from build123d import *

# Parameters (mm, degrees)
F10_W     = 100
F10_H     = 100
F14_DEPTH = 35
F13_W     = 70
F13_H     = 70
F15_DEPTH = 65
F16_T     = -5
F21_D     = 25.4


# Not quite as in the source:
# - the program builds the solid bodies; features that only make, move or delete a surface that nothing else refers to are left out


with BuildPart() as f14:
    # F10 (on offset) → F14 (new body, through all)
    with BuildSketch(Plane.XZ.offset(-406.68448)):
        with Locations((37.5531539321, 417.7168309689)):
            Rectangle(F10_W, F10_H)
    extrude(amount=-F14_DEPTH)

    # F13 (on offset) → F15 (join, through all)
    with BuildSketch(Plane.XZ.offset(-506.68448)):
        with Locations((37.5531539321, 417.7168309689)):
            Rectangle(F13_W, F13_H)
    extrude(amount=F15_DEPTH)

    # F16
    f16_openings = [f14.faces().sort_by_distance(p)[0] for p in [
        (37.553154, 406.68448, 417.716831),
    ]]
    offset(amount=F16_T, openings=f16_openings, kind=Kind.INTERSECTION)

    # F21 (through all)
    with Locations(Plane.XZ.offset(-441.68448)):
        with Locations((37.5531539321, 417.7168309689)):
            Hole(F21_D / 2)


solid = f14.part
Work out the finished part from the listing and answer in its coordinate system (mm). A direction names the side the tool comes from. Give positions to 0.01 mm unless a question says otherwise; leave off trailing zeros. Write each loop counter-clockwise with the first axis right and the second up, starting at its lowest first coordinate (ties: lowest second). Pieces come first, ordered by that corner, then holes. Notation, with made-up numbers: (69.5, -37) - (89.5, -37) arc R36 cw to (89.5, 2) - close; hole circle Ø3 at (-31.75, 41.5). An arc over 180 degrees is marked (long way). One line per item, written item: value. Start each with the question number.
1. Given pin 1 (6 mm diameter, centred on x = 32, y = 493, fed in from -Z); pin 2 (12 mm diameter, centred on y = 469.5, z = 419.5, fed in from +X); pin 3 (1 mm diameter, centred on x = 1.5, z = 383.5, fed in from +Y), each flat-ended and moving along its own axis, determine where each tip first touches the part or whether it passes through.
2. Find section B-B (x = 38). Write down the section's boundary in (y, z).
3. Find section D-D (x = 71). Write down the section's boundary in (y, z), then the cut area to 3 significant figures.
4. Find section A-A (y = 484). Write down the section's boundary in (x, z), then the cut area to 3 significant figures.
5. Consider probe 1 along Z at (x, y) = (33, 460); probe 2 along X at (y, z) = (460, 437); probe 3 along Z at (x, y) = (22, 419.5). Determine where each line is inside the solid, lowest interval first.
6. Find section C-C (z = 385). Write down the section's boundary in (x, y).
7. For a pull along Z with two mould halves and no side action, classify faces 6 (the flat face through (82.553, 421, 417)), 7 (the flat face through (34, 406.684, 370)), 8 (the flat face through (37, 424, 467.717)) as +Z half, -Z half, draft (parallel to the pull), parting line (faces both ways), or undercut.
8. For faces 1 (the flat face through (37, 475, 382.717)), 2 (the flat face through (2.553, 475, 417)), 3 (the flat face through (72.553, 475, 417)), 4 (the flat face through (87.553, 424, 417)), 5 (the flat face through (37, 470, 387.717)), determine the directions among +Z, -Z, +X, -X, +Y, -Y from which every point of the face is accessible in a straight line to the end or side of a thin tool.
Geometry results:
1. pin 1: z = 382.72
1. pin 2: x = 72.55
1. pin 3: y = 441.68
2. outline: (406.68, 367.72) - (441.68, 367.72) - (441.68, 382.72) - (506.68, 382.72) - (506.68, 405.02) - (501.68, 405.02) - (501.68, 387.72) - (436.68, 387.72) - (436.68, 372.72) - (406.68, 372.72) - close; (406.68, 462.72) - (436.68, 462.72) - (436.68, 447.72) - (501.68, 447.72) - (501.68, 430.41) - (506.68, 430.41) - (506.68, 452.72) - (441.68, 452.72) - (441.68, 467.72) - (406.68, 467.72) - close
3. outline: (406.68, 367.72) - (441.68, 367.72) - (441.68, 382.72) - (506.68, 382.72) - (506.68, 452.72) - (441.68, 452.72) - (441.68, 467.72) - (406.68, 467.72) - (406.68, 462.72) - (436.68, 462.72) - (436.68, 372.72) - (406.68, 372.72) - close
3. area: 5,350 mm2
4. outline: (2.55, 382.72) - (72.55, 382.72) - (72.55, 452.72) - (2.55, 452.72) - close; hole (7.55, 387.72) - (67.55, 387.72) - (67.55, 447.72) - (7.55, 447.72) - close
4. area: 1,300 mm2
5. probe 1: 382.72 to 387.72, 447.72 to 452.72
5. probe 2: 2.55 to 7.55, 67.55 to 72.55
5. probe 3: 367.72 to 372.72, 462.72 to 467.72
6. outline: (-12.45, 406.68) - (-7.45, 406.68) - (-7.45, 436.68) - (82.55, 436.68) - (82.55, 406.68) - (87.55, 406.68) - (87.55, 441.68) - (72.55, 441.68) - (72.55, 506.68) - (2.55, 506.68) - (2.55, 441.68) - (-12.45, 441.68) - close
7. face 6: undercut
7. face 7: draft
7. face 8: +Z half
8. face 1: -Z, +X, -X, +Y
8. face 2: +Z, -Z, -X, +Y
8. face 3: +Z, -Z, +X, +Y
8. face 4: +Z, -Z, +X, +Y, -Y
8. face 5: -Y
